Could you check a few things on this model? Use its own coordinates, in mm. Face numbers are marked on the shaded views. A direction names the side the tool comes from. Give positions to 0.01 mm unless a question says otherwise; leave off trailing zeros. Order: outer loops, then holes, each group sorted by start corner. A loop starts at its lowest first (then second) coordinate and runs counter-clockwise, first axis right, second up.
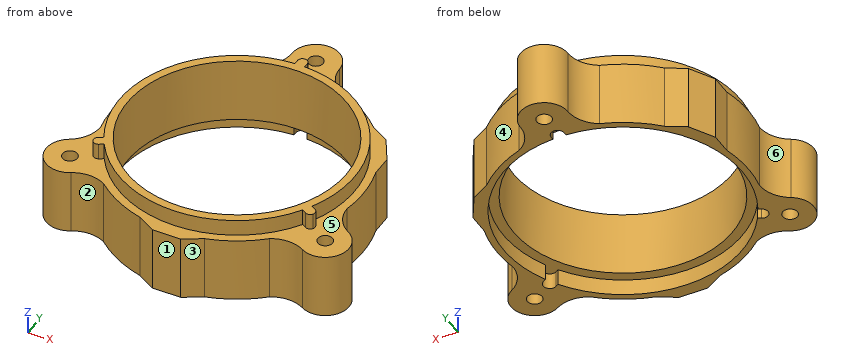
from build123d import *

# Parameters (mm, degrees)
F0_R     = 2.25
F0_R_2   = 33.35
F1_DEPTH = 20
F2_R     = 33.35
F3_DEPTH = 25
F5_DEPTH = 5
F6_R     = 1.49999
F8_DEPTH = 5
F9_SIZE  = 5


# Not quite as in the source:
# - a fillet or chamfer is up to 0.001 mm smaller than in the source, because OpenCascade refuses the exact size


with BuildPart() as f1:
    # F0 (on Top) → F1 (new body)
    with BuildSketch(Plane.XY):
        with BuildLine():
            ThreePointArc((-35.3461431703, -28.7786841774), (-30.3488782685, -27.4389385893), (-25.3508812473, -28.775950375))
            ThreePointArc((-25.3508812473, -28.775950375), (0, -38.35), (25.3508812473, -28.775950375))
            ThreePointArc((25.3508812473, -28.775950375), (30.3488782685, -27.4389385893), (35.3461431703, -28.7786841774))
            ThreePointArc((35.3461431703, -28.7786841774), (45.2498273477, -26.125), (42.5961431703, -16.2213158226))
            ThreePointArc((42.5961431703, -16.2213158226), (38.9372570055, -12.5634302623), (37.5961446665, -7.566531981))
            ThreePointArc((37.5961446665, -7.566531981), (33.2120742351, 19.175), (12.2452634191, 36.342482356))
            ThreePointArc((12.2452634191, 36.342482356), (8.588378737, 40.0023688516), (7.25, 45))
            ThreePointArc((7.25, 45), (0, 52.25), (-7.25, 45))
            ThreePointArc((-7.25, 45), (-8.588378737, 40.0023688516), (-12.2452634191, 36.342482356))
            ThreePointArc((-12.2452634191, 36.342482356), (-33.2120742351, 19.175), (-37.5961446665, -7.566531981))
            ThreePointArc((-37.5961446665, -7.566531981), (-38.9372570055, -12.5634302623), (-42.5961431703, -16.2213158226))
            ThreePointArc((-42.5961431703, -16.2213158226), (-45.2498273477, -26.125), (-35.3461431703, -28.7786841774))
        make_face()
        with Locations((-38.9711431703, -22.5)):
            Circle(F0_R, mode=Mode.SUBTRACT)
        with Locations((38.9711431703, -22.5)):
            Circle(F0_R, mode=Mode.SUBTRACT)
        Circle(F0_R_2, mode=Mode.SUBTRACT)
        with Locations((0, 45)):
            Circle(F0_R, mode=Mode.SUBTRACT)
    extrude(amount=F1_DEPTH)

    # F2 (on Top) → F3 (join)
    with BuildSketch(Plane.XY):
        Polygon((37.0225860118, -21.375), (37.0225860118, 21.375), (0, 42.75), (-37.0225860118, 21.375), (-37.0225860118, -21.375), (0, -42.75), align=None)
        Circle(F2_R, mode=Mode.SUBTRACT)
    extrude(amount=F3_DEPTH)

    # F4 (on face) → F5 (cut)
    with BuildSketch(Plane.XY.offset(25)):
        Polygon((37.0225860118, -21.375), (37.0225860118, 21.375), (0, 42.75), (-37.0225860118, 21.375), (-37.0225860118, -21.375), (0, -42.75), align=None)
        with BuildLine():
            ThreePointArc((-31.7698222916, -16.6102646446), (-31.0470107257, 17.925), (-1.5, 35.8186055005))
            Line((-1.5, 35.8186055005), (-1.5, 38.8186055005))
            Line((-1.5, 38.8186055005), (0, 38.8186055005))
            Line((0, 38.8186055005), (1.5, 38.8186055005))
            Line((1.5, 38.8186055005), (1.5, 35.8186055005))
            ThreePointArc((1.5, 35.8186055005), (31.0470107257, 17.925), (31.7698222916, -16.6102646446))
            Line((31.7698222916, -16.6102646446), (34.3678985029, -18.1102646446))
            Line((34.3678985029, -18.1102646446), (33.6178985029, -19.4093027502))
            Line((33.6178985029, -19.4093027502), (32.8678985029, -20.7083408559))
            Line((32.8678985029, -20.7083408559), (30.2698222916, -19.2083408559))
            ThreePointArc((30.2698222916, -19.2083408559), (0, -35.85), (-30.2698222916, -19.2083408559))
            Line((-30.2698222916, -19.2083408559), (-32.8678985029, -20.7083408559))
            Line((-32.8678985029, -20.7083408559), (-33.6178985029, -19.4093027502))
            Line((-33.6178985029, -19.4093027502), (-34.3678985029, -18.1102646446))
            Line((-34.3678985029, -18.1102646446), (-31.7698222916, -16.6102646446))
        make_face(mode=Mode.SUBTRACT)
    extrude(amount=-F5_DEPTH, mode=Mode.SUBTRACT)

    # F6 (radius 1.5 in the source; OpenCascade refuses exactly that, so slightly less here)
    f6_edges = [f1.edges().sort_by_distance(p)[0] for p in [
        (-32.867899, -20.708341, 22.5),
        (-34.367899, -18.110265, 22.5),
        (32.867899, -20.708341, 22.5),
        (34.367899, -18.110265, 22.5),
        (1.5, 38.818606, 22.5),
        (-1.5, 38.818606, 22.5),
    ]]
    fillet(f6_edges, radius=F6_R)

    # F7 (on Top) → F8 (cut)
    with BuildSketch(Plane.XY):
        with BuildLine():
            Line((-31.3188603972, -20.3913535578), (-30.4323380454, -19.8795196393))
            ThreePointArc((-30.4323380454, -19.8795196393), (0, -36.35), (30.4323380454, -19.8795196393))
            Line((30.4323380454, -19.8795196393), (31.3188603972, -20.3913535578))
            ThreePointArc((31.3188603972, -20.3913535578), (34.0509112048, -19.6593027502), (33.3188603972, -16.9272519427))
            Line((33.3188603972, -16.9272519427), (32.4323380454, -16.4154180242))
            ThreePointArc((32.4323380454, -16.4154180242), (31.4800234276, 18.175), (2, 36.2949376635))
            Line((2, 36.2949376635), (2, 37.3186055005))
            ThreePointArc((2, 37.3186055005), (0, 39.3186055005), (-2, 37.3186055005))
            Line((-2, 37.3186055005), (-2, 36.2949376635))
            ThreePointArc((-2, 36.2949376635), (-31.4800234276, 18.175), (-32.4323380454, -16.4154180242))
            Line((-32.4323380454, -16.4154180242), (-33.3188603972, -16.9272519427))
            ThreePointArc((-33.3188603972, -16.9272519427), (-34.0509112048, -19.6593027502), (-31.3188603972, -20.3913535578))
        make_face()
    extrude(amount=F8_DEPTH, mode=Mode.SUBTRACT)

    # F9
    f9_edges = [f1.edges().sort_by_distance(p)[0] for p in [
        (0, -42.75, 10),
        (37.022586, 21.375, 10),
        (-37.022586, 21.375, 10),
    ]]
    chamfer(f9_edges, length=F9_SIZE)


solid = f1.part
Item 1: Please list where these lines run through material, in increasing order: line 1 along Y through (x, z) = (0, 9); line 2 along X through (y, z) = (11.5, 6.25); line 3 along X through (y, z) = (0, 13).
Findings:
line 1: y = -40.25 to -33.35, 33.35 to 42.75, 47.25 to 52.25
line 2: x = -37.02 to -31.3, 31.3 to 37.02
line 3: x = -38.35 to -33.35, 33.35 to 38.35
Item 2: Imagine slicing it at C-C on x = -21. List the corners of the cut face in (y, z) for me.
Findings:
outline: (-32.09, 0) - (-29.67, 0) - (-29.67, 5) - (-25.91, 5) - (-25.91, 25) - (-29.06, 25) - (-29.06, 20) - (-32.09, 20) - close; (25.91, 5) - (29.67, 5) - (29.67, 0) - (32.09, 0) - (32.09, 20) - (29.06, 20) - (29.06, 25) - (25.91, 25) - close
Item 3: Imagine slicing it at A-A on y = 0. List the corners of the cut face in (x, z) for me.
Findings:
outline: (-38.35, 0) - (-36.35, 0) - (-36.35, 5) - (-33.35, 5) - (-33.35, 25) - (-35.85, 25) - (-35.85, 20) - (-38.35, 20) - close; (33.35, 5) - (36.35, 5) - (36.35, 0) - (38.35, 0) - (38.35, 20) - (35.85, 20) - (35.85, 25) - (33.35, 25) - close
Item 4: Imagine slicing it at B-B on z = 6.25. List the corners of the cut face in (x, y) for me (3 decimals).
Findings:
outline: (-42.596, -16.221) arc R7.25 ccw to (-35.346, -28.779) arc R10 cw to (-25.351, -28.776) arc R38.35 ccw to (-9.849, -37.064) - (-4.33, -40.25) - (4.33, -40.25) - (9.849, -37.064) arc R38.35 ccw to (25.351, -28.776) arc R10 cw to (35.346, -28.779) arc R7.25 ccw to (42.596, -16.221) arc R10 cw to (37.596, -7.567) arc R38.35 ccw to (37.023, 10.003) - (37.023, 16.375) - (32.692, 23.875) - (27.174, 27.061) arc R38.35 ccw to (12.245, 36.342) arc R10 cw to (7.25, 45) arc R7.25 ccw to (-7.25, 45) arc R10 cw to (-12.245, 36.342) arc R38.35 ccw to (-27.174, 27.061) - (-32.692, 23.875) - (-37.023, 16.375) - (-37.023, 10.003) arc R38.35 ccw to (-37.596, -7.567) arc R10 cw to start; hole circle Ø4.5 at (-38.971, -22.5); hole circle Ø66.7 at (0, 0); hole circle Ø4.5 at (0, 45); hole circle Ø4.5 at (38.971, -22.5)
Item 5: For pin 1 (7 mm diameter, centred on x = 38.97, y = -22.5, fed in from +Z); pin 2 (6 mm diameter, centred on x = 29.5, y = -19.5, fed in from -Z); pin 3 (1.5 mm diameter, centred on y = -9, z = 5.5, fed in from +X); pin 4 (1 mm diameter, centred on x = -10.5, z = 15.5, fed in from +Y), each with a flat end and sliding along its axis, tell me the tip position at first contact or that it passes through.
Findings:
pin 1: stops at z = 20
pin 2: stops at z = 0
pin 3: stops at x = 37.84
pin 4: stops at y = 38.11
Item 6: For the marked faces 4, 5 and 6, which set-ups out of +Z, -Z, +X, -X, +Y, -Y let a thin tool reach every point of the face, with its end or its side?
Findings:
face 4: +Z, -Z, +X, +Y
face 5: +Z
face 6: +Z, -Z, -X
Item 7: We'd pull the mould along X, two halves only. Please class the marked faces 1, 2 and 3: +X half, -X half, draft (parallel to the pull), parting line (faces both ways), or undercut.
Findings:
face 1: draft
face 2: undercut
face 3: +X half
